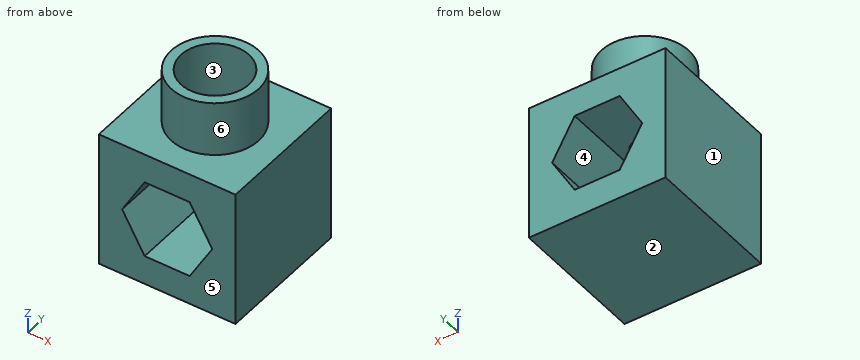
```python
from build123d import *

# Parameters (mm, degrees)
F0_W     = 150
F0_H     = 150
F1_DEPTH = 150
F2_R     = 47.966338
F2_R_2   = 37.217605
F3_DEPTH = 60
F5_DEPTH = 150.001
F6_R     = 14.151474
F7_DEPTH = 32.145534


with BuildPart() as f1:
    # F0 (on Front) → F1 (new body)
    with BuildSketch(Plane.XZ):
        Rectangle(F0_W, F0_H)
    extrude(amount=F1_DEPTH)

    # F2 (on face) → F3 (join)
    with BuildSketch(Plane.XY.offset(75)):
        with Locations((0, -75)):
            Circle(F2_R)
        with Locations((0, -75)):
            Circle(F2_R_2, mode=Mode.SUBTRACT)
    extrude(amount=F3_DEPTH)

    # F4 (on face) → F5 (cut, through all)
    with BuildSketch(Plane.XZ.offset(150)):
        Polygon((49.484075, 0), (24.742038, 42.854466), (-24.742038, 42.854466), (-49.484075, 0), (-24.742038, -42.854466), (24.742038, -42.854466), align=None)
    extrude(amount=-F5_DEPTH, mode=Mode.SUBTRACT)

    # F6 (on face) → F7 (cut, through all)
    with BuildSketch(Plane.XY.offset(75)):
        with Locations((0, -75)):
            Circle(F6_R)
    extrude(amount=-F7_DEPTH, mode=Mode.SUBTRACT)


solid = f1.part
```
Geometry check sheet. Reference: the model listing, model coordinates, mm. Face numbers are marked on the shaded views. A direction names the side the tool comes from. Give positions to 0.01 mm unless a question says otherwise; leave off trailing zeros. Write each loop counter-clockwise with the first axis right and the second up, starting at its lowest first coordinate (ties: lowest second). Pieces come first, ordered by that corner, then holes.
1) Gauge pin test, flat ends, axial feed: pin 1 (8 mm diameter, centred on x = -29.5, y = -78.5, fed in from +Z); pin 2 (10 mm diameter, centred on x = -41, z = 7, fed in from -Y); pin 3 (6 mm diameter, centred on y = -53.5, z = 99.5, fed in from -X). Record the tip position at first contact, or that the pin passes through.
2) Section check B-B, the plane x = 0. Record the boundary of the cut face in (y, z).
3) Material ranges on L1, parallel to Z at x = -10.5, y = -106; L2, parallel to Y at x = 0, z = 89; L3, parallel to Y at x = 0, z = 51, recorded low to high.
4) Section check C-C, the plane z = 61.5. Record the boundary of the cut face in (x, y), and give its area (3 significant figures).
5) Section check D-D, the plane y = -75. Record the boundary of the cut face in (x, z).
6) Release check for a two-part mould opening along X. For the marked faces 1, 2 and 3 record: pulls with the +X half, pulls with the -X half, needs draft (parallel to the pull), parting line crosses it, or undercut.
7) Access from +Z, -Z, +X, -X, +Y, -Y to the whole of each face (thin tool, end or side, straight path). Record for the marked faces 4, 5 and 6.
8) Section check A-A, the plane y = -19.5. Record the boundary of the cut face in (x, z), and give its area (3 significant figures).
Computed:
1. pin 1: stops at z = 75
1. pin 2: stops at y = -150
1. pin 3: stops at x = -44.26
2. outline: (-150, -75) - (0, -75) - (0, -42.85) - (-150, -42.85) - close; (-150, 42.85) - (-89.15, 42.85) - (-89.15, 75) - (-112.22, 75) - (-112.22, 135) - (-122.97, 135) - (-122.97, 75) - (-150, 75) - close; (-60.85, 42.85) - (0, 42.85) - (0, 75) - (-27.03, 75) - (-27.03, 135) - (-37.78, 135) - (-37.78, 75) - (-60.85, 75) - close
3. L1: z = -75 to -42.85, 42.85 to 75
3. L2: y = -122.97 to -112.22, -37.78 to -27.03
3. L3: y = -150 to -89.15, -60.85 to 0
4. outline: (-75, -150) - (75, -150) - (75, 0) - (-75, 0) - close; hole circle Ø28.3 at (0, -75)
4. area: 21,900 mm2
5. outline: (-75, -75) - (75, -75) - (75, 75) - (47.97, 75) - (47.97, 135) - (37.22, 135) - (37.22, 75) - (14.15, 75) - (14.15, 42.85) - (24.74, 42.85) - (49.48, 0) - (24.74, -42.85) - (-24.74, -42.85) - (-49.48, 0) - (-24.74, 42.85) - (-14.15, 42.85) - (-14.15, 75) - (-37.22, 75) - (-37.22, 135) - (-47.97, 135) - (-47.97, 75) - (-75, 75) - close
6. face 1: pulls with the -X half
6. face 2: needs draft
6. face 3: undercut
7. face 4: +Y, -Y
7. face 5: +Z, -Z, +X, -X, -Y
7. face 6: +Z
8. outline: (-75, -75) - (75, -75) - (75, 75) - (-75, 75) - close; hole (-49.48, 0) - (-24.74, -42.85) - (24.74, -42.85) - (49.48, 0) - (24.74, 42.85) - (-24.74, 42.85) - close
8. area: 16,100 mm2
